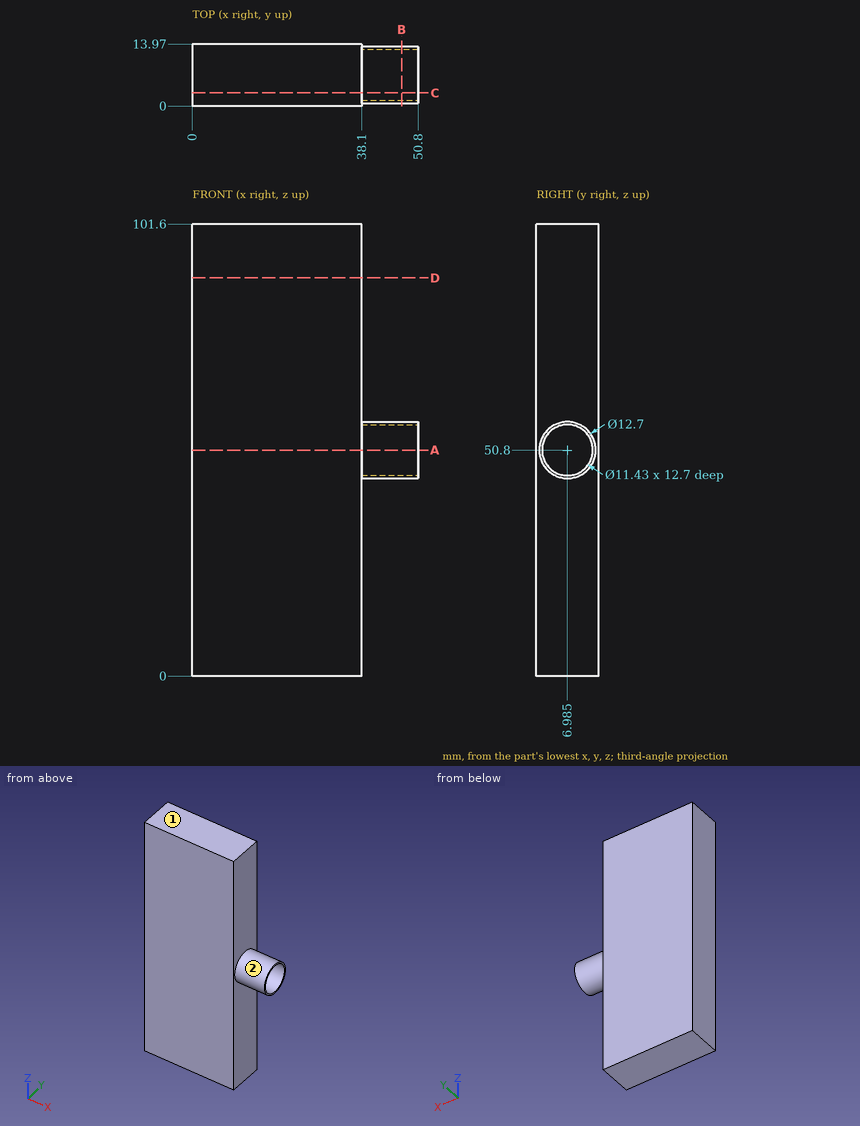
Drawing for the job (mm, zero at the part's lowest x, y, z). A direction names the side the tool comes from. Round coordinates to 2 decimals unless told otherwise and drop trailing zeros. Loops run counter-clockwise (first coordinate to the right, second up) from the corner with the lowest first, then second, coordinate; pieces in that order, holes last. Notation, with made-up numbers: (52, -30.5) - (86, -30.5) arc R30 ccw to (86, -5.5) - close; hole circle Ø11 at (-29.75, 39.25). An arc over 180 degrees is marked (long way). Write each question's results on one line, items separated by ' | '.
(1) Saw through at A-A, the plane z = 50.8. List the corners of the cut face in (x, y) (3 decimals).
Answer below:
outline: (0, 0) - (38.1, 0) - (38.1, 0.635) - (50.8, 0.635) - (50.8, 1.27) - (38.1, 1.27) - (38.1, 12.7) - (50.8, 12.7) - (50.8, 13.335) - (38.1, 13.335) - (38.1, 13.97) - (0, 13.97) - close
(2) Saw through at D-D, the plane z = 89.5. List the corners of the cut face in (x, y), then the cut area to 3 significant figures.
Answer below:
outline: (0, 0) - (38.1, 0) - (38.1, 13.97) - (0, 13.97) - close | area: 532 mm^2
(3) Pin check, flat tips, straight feed: pin 1 (1.5 mm diameter, centred on y = 2.5, z = 19, fed in from -X); pin 2 (3 mm diameter, centred on x = 44, y = 12, fed in from -Z). Stop position of each tip, or through.
Answer below:
pin 1: stops at x = 0 | pin 2: stops at z = 45.51
(4) Saw through at B-B, the plane x = 47. List the corners of the cut face in (y, z) (3 decimals), then the cut area to 3 significant figures.
Answer below:
outline: circle Ø12.7 at (6.985, 50.8); hole circle Ø11.43 at (6.985, 50.8) | area: 24.1 mm^2
(5) 3-axis set-ups, long thin cutter, end or side, ignore diameter. For the marked faces 1 and 2: which of +Z, -Z, +X, -X, +Y, -Y reach the whole face in a straight line?
Answer below:
face 1: +Z, +X, -X, +Y, -Y | face 2: +X
(6) Wall check: L1, parallel to X at y = 10.25, z = 67; L2, parallel to Z at x = 46, y = 5.5; L3, parallel to Z at x = 46.5, y = 2.5. Give the ranges that are in metal, low to high.
Answer below:
L1: x = 0 to 38.1 | L2: z = 44.63 to 45.28, 56.32 to 56.97 | L3: z = 46.3 to 47.26, 54.34 to 55.3
(7) Saw through at C-C, the plane y = 3. List the corners of the cut face in (x, z).
Answer below:
outline: (0, 0) - (38.1, 0) - (38.1, 45.86) - (50.8, 45.86) - (50.8, 46.7) - (38.1, 46.7) - (38.1, 54.9) - (50.8, 54.9) - (50.8, 55.74) - (38.1, 55.74) - (38.1, 101.6) - (0, 101.6) - close
